The model under review builds one solid part; all positions refer to its coordinate system, in mm. A direction names the side the tool comes from. Round coordinates to 2 decimals unless told otherwise and drop trailing zeros. Write each loop counter-clockwise with the first axis right and the second up, starting at its lowest first coordinate (ties: lowest second). Pieces come first, ordered by that corner, then holes.
Item 1: To check wall thickness, follow L1, parallel to X at y = 343.5, z = 3; L2, parallel to Y at x = 110, z = 2; L3, parallel to X at y = 362, z = 0.75. State the ranges of each line that lie inside material, in increasing order.
Item 2: Draft analysis for pull direction Y (two halves, no side actions). For faces 3 (the face through (85.743, 355.226, 6.261)), 4 (the face through (117, 263.176, 6)), 5 (the face through (142.737, 271.624, 3.519)), 6 (the face through (181.397, 363, 6)), state which applies: +Y half, -Y half, draft (parallel to the pull), parting line (faces both ways), or undercut.
Item 3: Add section B-B (z = 3.75). State how many separate pieces and enclosed holes the cut face has, plus the area to 3 significant figures.
Item 4: Add section C-C (x = 144.5). Give the boundary of the cut face in (y, z).
Item 5: Clearance check with a flat-ended pin moving along its axis: pin 1 Ø5.5 at (x, y) = (91.5, 364.5) entering from -Z. State where the tip first meets the part, or that it passes through.
Item 6: Add section A-A (x = 74). Give the boundary of the cut face in (y, z).
Item 7: Machinability: for faces 1 (the face through (117, 366, 0)), 2 (the face through (74.66, 342.97, 3.52)), which of the approach directions +Z, -Z, +X, -X, +Y, -Y give a long, thin tool a straight path to every point of the face, cutting with its end or side? Answer none if there is none.
```python
from build123d import *

# Parameters (mm, degrees)
SKETCH1_W           = 126.991036612
SKETCH1_H           = 203.20170097
SKETCH1_R           = 3.5687
SKETCH1_R_2         = 3.175
SKETCH1_R_3         = 3.556
BOSS_EXTRUDE1_DEPTH = 12.7
SKETCH2_R           = 5.5499
CUT_EXTRUDE1_DEPTH  = 7.1374


with BuildPart() as part:
    # Sketch1 → Boss-Extrude1 (new body)
    with BuildSketch(Plane.XY):
        with Locations((117.901436969, 364.776968974)):
            Rectangle(SKETCH1_W, SKETCH1_H)
        with Locations((163.258479874, 294.508127154)):
            Circle(SKETCH1_R, mode=Mode.SUBTRACT)
        with Locations((145.297967632, 276.547614912)):
            Circle(SKETCH1_R, mode=Mode.SUBTRACT)
        with Locations((91.416430905, 366.350176123)):
            Circle(SKETCH1_R, mode=Mode.SUBTRACT)
        with Locations((73.455918663, 348.389663881)):
            Circle(SKETCH1_R, mode=Mode.SUBTRACT)
        with Locations((86.155918663, 428.277819459)):
            Circle(SKETCH1_R_2, mode=Mode.SUBTRACT)
        with Locations((111.555918663, 428.277819459)):
            Circle(SKETCH1_R_2, mode=Mode.SUBTRACT)
        with Locations((86.155918663, 352.077819459)):
            Circle(SKETCH1_R_2, mode=Mode.SUBTRACT)
        with Locations((111.555918663, 352.077819459)):
            Circle(SKETCH1_R_3, mode=Mode.SUBTRACT)
    extrude(amount=BOSS_EXTRUDE1_DEPTH)

    # Sketch2 → Cut-Extrude1 (cut)
    with BuildSketch(Plane(origin=(0, 0, 0), x_dir=(-1, 0, 0), z_dir=(0, 0, -1))):
        with Locations((-91.416430905, 366.350176123)):
            Circle(SKETCH2_R)
        with Locations((-73.455918663, 348.389663881)):
            Circle(SKETCH2_R)
        with Locations((-163.258479874, 294.508127154)):
            Circle(SKETCH2_R)
        with Locations((-145.297967632, 276.547614912)):
            Circle(SKETCH2_R)
    extrude(amount=-CUT_EXTRUDE1_DEPTH, mode=Mode.SUBTRACT)


solid = part.part
```
Numbers:
1. L1: x = 54.41 to 70.83, 76.08 to 181.4
1. L2: y = 263.18 to 348.88, 355.28 to 425.51, 431.05 to 466.38
1. L3: x = 54.41 to 87.97, 94.86 to 181.4
2. face 3: undercut
2. face 4: -Y half
2. face 5: undercut
2. face 6: draft
3. separate pieces: 1
3. enclosed holes: 8
3. area: 25,300 mm2
4. outline: (263.18, 0) - (271.06, 0) - (271.06, 7.14) - (273.07, 7.14) - (273.07, 12.7) - (263.18, 12.7) - close; (280.03, 7.14) - (282.04, 7.14) - (282.04, 0) - (466.38, 0) - (466.38, 12.7) - (280.03, 12.7) - close
5. pin 1: stops at z = 7.14
6. outline: (263.18, 0) - (342.87, 0) - (342.87, 7.14) - (344.86, 7.14) - (344.86, 12.7) - (263.18, 12.7) - close; (351.92, 7.14) - (353.91, 7.14) - (353.91, 0) - (466.38, 0) - (466.38, 12.7) - (351.92, 12.7) - close
7. face 1: -Z, +X, -X, +Y, -Y
7. face 2: -Z
